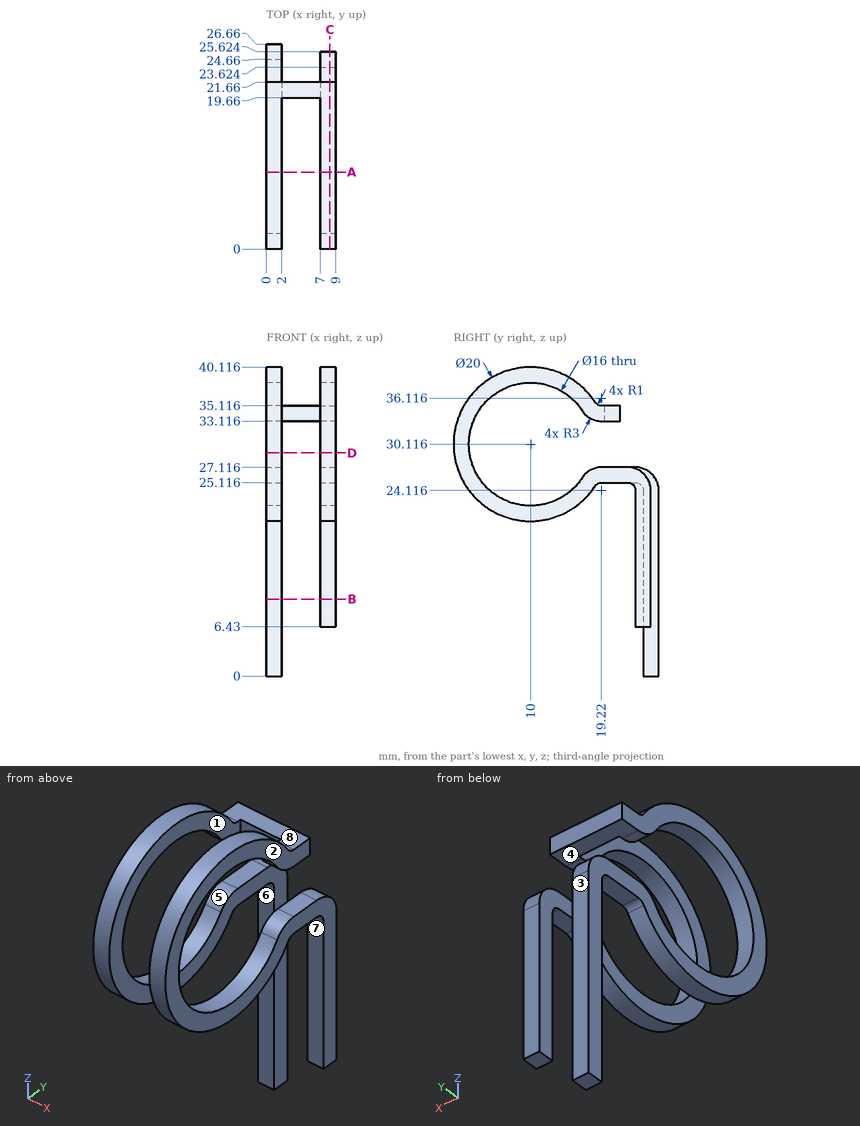
Geometry check sheet. Reference: drawing and pictorial views, mm from the part's lowest x, y, z. A direction names the side the tool comes from. Round coordinates to 2 decimals unless told otherwise and drop trailing zeros. Order: outer loops, then holes, each group sorted by start corner. A loop starts at its lowest first (then second) coordinate and runs counter-clockwise, first axis right, second up. Notation, with made-up numbers: (81, 32.25) -> (100, 32.25) arc R15 ccw to (100, 40.25) -> close; hole circle Ø1 at (50, 33). An arc over 180 degrees is marked (long way). One line per item, written item: value. Start each with the question number.
Q1. Cross-section at A-A (y = 10). Record the boundary of the cut face in (x, z) (1 decimal), and give its area (3 significant figures).
Q2. Thickness scan on line 1 (X direction, y = 19, z = 27); line 2 (Z direction, x = 1, y = 21) (1 decimal); line 3 (Z direction, x = 8.25, y = 10) (1 decimal). Record the ranges inside material, lowest first.
Q3. Cross-section at D-D (z = 29). Record the boundary of the cut face in (x, y).
Q4. Cross-section at B-B (z = 10). Record the boundary of the cut face in (x, y).
Q5. Set-up check for the marked faces 4, 5, 6, 7 and 8: record each of +Z, -Z, +X, -X, +Y, -Y from which the full face is reachable in a straight line by a thin tool's end or side.
Q6. Cross-section at C-C (x = 8.25). Record the boundary of the cut face in (y, z) (1 decimal).
Q7. Mould release check, pull along X, two halves, no side actions. Record for the marked faces 1, 2 and 3: pulls with the +X half, pulls with the -X half, needs draft (parallel to the pull), parting line crosses it, or undercut.
Q8. Gauge pin test, flat ends, axial feed: pin 1 Ø1.6 at (x, z) = (4.5, 34) entering from +Y; pin 2 Ø1.2 at (x, y) = (5.5, 20) entering from -Z; pin 3 Ø1 at (x, y) = (1.5, 21.5) entering from +Z. Record the tip position at first contact, or that the pin passes through.
Completed:
1. outline: (0, 20.1) -> (2, 20.1) -> (2, 22.1) -> (0, 22.1) -> close; (0, 38.1) -> (2, 38.1) -> (2, 40.1) -> (0, 40.1) -> close; (7, 20.1) -> (9, 20.1) -> (9, 22.1) -> (7, 22.1) -> close; (7, 38.1) -> (9, 38.1) -> (9, 40.1) -> (7, 40.1) -> close
1. area: 16.0 mm²
2. line 1: x = 0 to 2, 7 to 9
2. line 2: z = 25.1 to 27.1, 33.1 to 35.1
2. line 3: z = 20.1 to 22.1, 38.1 to 40.1
3. outline: (0, 0.06) -> (2, 0.06) -> (2, 2.08) -> (0, 2.08) -> close; (7, 0.06) -> (9, 0.06) -> (9, 2.08) -> (7, 2.08) -> close
4. outline: (0, 24.66) -> (2, 24.66) -> (2, 26.66) -> (0, 26.66) -> close; (7, 23.62) -> (9, 23.62) -> (9, 25.62) -> (7, 25.62) -> close
5. face 4: +X, -X, +Y
5. face 5: +X, -X
5. face 6: -Z, -X
5. face 7: -Z, +X, -X
5. face 8: +Z, +X, -X, +Y
6. outline: (16.7, 25.8) arc R8 cw (long way) to (16.7, 34.5) arc R3 ccw to (19.2, 33.1) -> (21.7, 33.1) -> (21.7, 35.1) -> (19.2, 35.1) arc R1 cw to (18.4, 35.6) arc R10 ccw (long way) to (18.4, 24.7) arc R1 cw to (19.2, 25.1) -> (22.6, 25.1) arc R1 cw to (23.6, 24.1) -> (23.6, 6.4) -> (25.6, 6.4) -> (25.6, 24.1) arc R3 ccw to (22.6, 27.1) -> (19.2, 27.1) arc R3 ccw to start
7. face 1: undercut
7. face 2: pulls with the +X half
7. face 3: needs draft
8. pin 1: stops at y = 21.66
8. pin 2: stops at z = 33.12
8. pin 3: stops at z = 35.12
